Part model, mm, in its own coordinate system. Coordinates: 2 decimals unless noted, no trailing zeros. Loops run counter-clockwise (first coordinate to the right, second up) from the corner with the lowest first, then second, coordinate; pieces in that order, holes last. Notation, with made-up numbers: M 2.25,41 L 29.25,41 A16 cw 29.25,47 Z; hole C 57,74.25 d1. An arc over 180 degrees is marked long. Answer as CSV lines item,"result". Start each with the question number.
Autodesk Inventor part; units mm, degrees
ref_plane "YZ Plane" through (0, 0, 0) normal (1, 0, 0) x (0, 1, 0)
ref_plane "XZ Plane" through (0, 0, 0) normal (0, 1, 0) x (-1, 0, 0)
ref_plane "XY Plane" through (0, 0, 0) normal (0, 0, 1) x (1, 0, 0)
sketch "Sketch1" plane through (0, 0, 0) normal (0, 0, 1) x (1, 0, 0)
  line L0 (-158.3346, -22.9633) -> (-158.3346, -15.0367)
  arc A0 (-32.2589, 3) -> (-35, 2.3373) centre (-32.2589, -3) ccw
  line L1 (-35, 2.3373) -> (-35, -5)
  line L2 (0, -5) -> (-35, -5)
  line L3 (0, 3) -> (0, -5)
  line L4 (0, 3) -> (-32.2589, 3)
  circle A1 centre (-8, -1) radius 2
  circle A2 centre (-24, -1) radius 2
  line L5 (-158.3346, -19) -> (0, -19)
  line L6 (-64, 3) -> (-56, 3)
  line L7 (-60, 3) -> (-60, 13)
  line L8 (-60, 13) -> (50, 13)
  line L9 (-32.2589, 3) -> (-32.2589, -5)
  line L10 (50, 13) -> (50, -19)
  line L11 (50, -19) -> (40, -19)
  line L12 (40, -19) -> (30, -19)
  line L13 (20, -15) -> (40, -15)
  line L14 (40, -15) -> (40, -23)
  line L15 (40, -23) -> (20, -23)
  line L16 (20, -23) -> (20, -15)
  line L17 (20, -15) -> (40, -23) construction
  line L18 (40, -15) -> (20, -23) construction
  line L19 (0, 3) -> (40, -15)
  line L20 (30, -19) -> (24, -19)
  circle A3 centre (24, -19) radius 1.5
  line L21 (30, -19) -> (36, -19)
  circle A4 centre (36, -19) radius 1.5
  line L22 (-32.2589, -5) -> (20, -23)
  point P0 (0, 0)
  dimension "d0" = 10
  dimension "d1" = 110
  dimension "d2" = 32
  dimension "d3" = 10
  dimension "d4" = 10
  dimension "d5" = 20
  dimension "d6" = 8
  dimension "d7" = 6
  dimension "d8" = 3
  dimension "d9" = 6
  dimension "d10" = 3
extrude "Extrusion1" add sketch "Sketch1" along normal blind 2 contours L4 L3 L2 L9 | L19 L13 L16 L22 L2 L3 | L14 L15 L16 L13
sketch "Sketch3" plane through (0, 0, 0) normal (0, 0, -1) x (-1, 0, 0)
  line L0 (0, 3) -> (32.2589, 3)
  line L1 (-40, -15) -> (0, 3)
  line L2 (-40, -23) -> (-40, -15)
  line L3 (-20, -23) -> (-40, -23)
  line L4 (32.2589, -5) -> (-20, -23)
  line L5 (32.2589, 3) -> (32.2589, -5)
  circle A0 centre (-36, -19) radius 1.5
  circle A1 centre (-24, -19) radius 1.5
  circle A2 centre (24, -1) radius 2
  circle A3 centre (8, -1) radius 2
  circle A4 centre (8, -1) radius 1.5
  circle A5 centre (24, -1) radius 1.5
  point P0 (0, 0)
  dimension "d23" = 3
  dimension "d24" = 3
extrude "Extrusion3" add sketch "Sketch3" against normal blind 2 contours A2 | A3
sketch "Sketch4" plane through (0, 0, 2) normal (0, 0, 1) x (1, 0, 0)
  circle A0 centre (-24, -1) radius 1.5
  circle A1 centre (-8, -1) radius 1.5
  line L0 (-32.2589, 3) -> (-32.2589, -5)
  line L1 (-32.2589, -5) -> (20, -23)
  line L2 (20, -23) -> (40, -23)
  line L3 (40, -23) -> (40, -15)
  line L4 (40, -15) -> (0, 3)
  line L5 (0, 3) -> (-32.2589, 3)
  circle A2 centre (36, -19) radius 1.5
  circle A3 centre (24, -19) radius 1.5
  circle A4 centre (-8, -1) radius 1.5
  line L6 (-8, -1) -> (24, -19)
  line L7 (1.0274, -6.0779) -> (14.9726, -13.9221) construction
  line L8 (-0.0757, -8.039) -> (13.8695, -15.8831)
  line L9 (16.0757, -11.961) -> (2.1305, -4.1169)
  arc A5 (2.1305, -4.1169) -> (-0.0757, -8.039) centre (1.0274, -6.0779) ccw
  arc A6 (13.8695, -15.8831) -> (16.0757, -11.961) centre (14.9726, -13.9221) ccw
  point P0 (0, 0)
  point P1 (8, -10)
  dimension "d27" = 8
  dimension "d28" = 4.5
extrude "Extrusion4" cut sketch "Sketch4" against normal blind 10 contours A5 L9 A6 L6 | L6 A6 L8 A5
properties part number "arm_2"
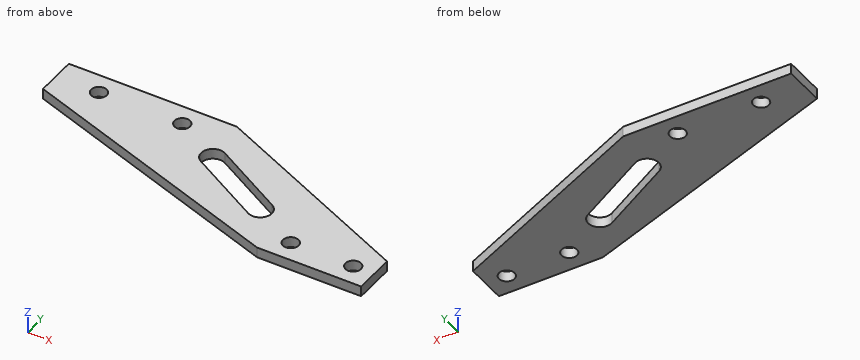
Q1. Slice it at C-C, the plane y = -19. Write the cut outline in (x, z).
Q2. Slice it at A-A, the plane x = 36. Write the cut outline in (y, z).
Q3. Slice it at B-B, the plane z = 1.3. Write the cut outline in (x, y).
Q4. Slice it at D-D, the plane x = 24. Write the cut outline in (y, z).
Q5. Wall check: L1, parallel to X at y = -0.25, z = 1.65; L2, parallel to X at y = -0.5, z = 0.2; L3, parallel to Y at x = 24, z = 1.1. Give the ranges that are in metal, low to high.
Solved:
1,outline,"M 8.39,0 L 22.5,0 L 22.5,2 L 8.39,2 Z; M 25.5,0 L 34.5,0 L 34.5,2 L 25.5,2 Z; M 37.5,0 L 40,0 L 40,2 L 37.5,2 Z"
2,outline,"M -23,0 L -20.5,0 L -20.5,2 L -23,2 Z; M -17.5,0 L -13.2,0 L -13.2,2 L -17.5,2 Z"
3,outline,"M -32.26,-5 L 20,-23 L 40,-23 L 40,-15 L 0,3 L -32.26,3 Z; hole C -24,-1 d3; hole C -8,-1 d3; hole M -0.08,-8.04 L 13.87,-15.88 A2.25 ccw 16.08,-11.96 L 2.13,-4.12 A2.25 ccw Z; hole C 24,-19 d3; hole C 36,-19 d3"
4,outline,"M -23,0 L -20.5,0 L -20.5,2 L -23,2 Z; M -17.5,0 L -7.8,0 L -7.8,2 L -17.5,2 Z"
5,L1,"x = -32.26 to -25.3, -22.7 to -9.3, -6.7 to 7.22"
5,L2,"x = -32.26 to -25.41, -22.59 to -9.41, -6.59 to 7.78"
5,L3,"y = -23 to -20.5, -17.5 to -7.8"
